Here's how the part is built. I have some questions about the finished solid (model axes, mm). A direction names the side the tool comes from. Give positions to 0.01 mm unless a question says otherwise; leave off trailing zeros. Write each loop counter-clockwise with the first axis right and the second up, starting at its lowest first coordinate (ties: lowest second). Pieces come first, ordered by that corner, then holes. Notation, with made-up numbers: (40, 58.5) - (70, 58.5) arc R36 ccw to (70, 92.5) - close; hole circle Ø11 at (-9, 82). An arc over 180 degrees is marked (long way). One line per item, written item: value. Start each with the question number.
1) I'm going to push a flat-ended pin straight in: P1, Ø4.5, axis at y = 0, z = 76.2, coming from the -X side. Where does the tip first touch, or does it pass through?
2) Imagine slicing it at A-A on z = -157.5. Write out the boundary of the cut face in (x, y) (3 decimals), plus the area to 3 significant figures.
3) Please list where these lines run through material, in increasing order: L1, parallel to Y at x = 8.5, z = 11.5 (3 decimals); L2, parallel to X at y = -7.25, z = -201 (3 decimals); L3, parallel to Y at x = -24, z = -76. Write a range as [from, to].
4) We'd pull the mould along Y, two halves only. Please class faces 1 (the flat face through (-22.225, 0, 3)), 2 (the flat face through (0, 9.525, 3)), 3 (the flat face through (0, 10, 222.25)), 4 (the flat face through (0, -12.7, 3)): +Y half, -Y half, draft (parallel to the pull), parting line (faces both ways), or undercut.
5) On a 3-axis mill with a long thin cutter (end or side, diameter ignored), from which of +Z, -Z, +X, -X, +Y, -Y can I reach the whole of each face in a straight line? I mean faces 5 (the flat face through (-25.4, 0, 3)), 6 (the flat face through (22.225, 0, 3)). Say none if no direction works.
from build123d import *

# Parameters (mm, degrees)
SKETCH1_W           = 50.8
SKETCH1_H           = 25.4
SKETCH1_W_2         = 44.45
SKETCH1_H_2         = 19.05
BOSS_EXTRUDE1_DEPTH = 222.25
SKETCH3_R           = 2.15265
SKETCH3_R_2         = 2.159
CUT_EXTRUDE2_DEPTH  = 51.8
SKETCH4_R           = 2.4892
CUT_EXTRUDE3_DEPTH  = 51.8
SKETCH5_R           = 2.4892
CUT_EXTRUDE4_DEPTH  = 26.4


with BuildPart() as part:
    # Sketch1 → Boss-Extrude1 (new body, symmetric)
    with BuildSketch(Plane.XY):
        Rectangle(SKETCH1_W, SKETCH1_H)
        Rectangle(SKETCH1_W_2, SKETCH1_H_2, mode=Mode.SUBTRACT)
    extrude(amount=BOSS_EXTRUDE1_DEPTH, both=True)

    # Sketch3 → Cut-Extrude2 (cut, through all)
    with BuildSketch(Plane(origin=(25.4, 0, 0), x_dir=(0, 0, -1), z_dir=(1, 0, 0))):
        with Locations((-215.9, 0)):
            Circle(SKETCH3_R)
        with Locations((-190.5, 0)):
            Circle(SKETCH3_R)
        with Locations((-165.1, 0)):
            Circle(SKETCH3_R)
        with Locations((215.9, 0)):
            Circle(SKETCH3_R_2)
        with Locations((190.5, 0)):
            Circle(SKETCH3_R_2)
        with Locations((165.1, 0)):
            Circle(SKETCH3_R_2)
    extrude(amount=-CUT_EXTRUDE2_DEPTH, mode=Mode.SUBTRACT)

    # Sketch4 → Cut-Extrude3 (cut, through all)
    with BuildSketch(Plane(origin=(25.4, 0, 0), x_dir=(0, 0, -1), z_dir=(1, 0, 0))):
        with Locations((-139.7, 0)):
            Circle(SKETCH4_R)
        with Locations((-127, 0)):
            Circle(SKETCH4_R)
        with Locations((-114.3, 0)):
            Circle(SKETCH4_R)
        with Locations((-101.6, 0)):
            Circle(SKETCH4_R)
        with Locations((-88.9, 0)):
            Circle(SKETCH4_R)
        with Locations((-76.2, 0)):
            Circle(SKETCH4_R)
        with Locations((-63.5, 0)):
            Circle(SKETCH4_R)
        with Locations((-50.8, 0)):
            Circle(SKETCH4_R)
        with Locations((-38.1, 0)):
            Circle(SKETCH4_R)
        with Locations((-25.4, 0)):
            Circle(SKETCH4_R)
        with Locations((-12.7, 0)):
            Circle(SKETCH4_R)
        Circle(SKETCH4_R)
        with Locations((12.7, 0)):
            Circle(SKETCH4_R)
        with Locations((25.4, 0)):
            Circle(SKETCH4_R)
        with Locations((38.1, 0)):
            Circle(SKETCH4_R)
        with Locations((50.8, 0)):
            Circle(SKETCH4_R)
        with Locations((63.5, 0)):
            Circle(SKETCH4_R)
        with Locations((76.2, 0)):
            Circle(SKETCH4_R)
        with Locations((88.9, 0)):
            Circle(SKETCH4_R)
        with Locations((101.6, 0)):
            Circle(SKETCH4_R)
        with Locations((114.3, 0)):
            Circle(SKETCH4_R)
        with Locations((127, 0)):
            Circle(SKETCH4_R)
        with Locations((139.7, 0)):
            Circle(SKETCH4_R)
    extrude(amount=-CUT_EXTRUDE3_DEPTH, mode=Mode.SUBTRACT)

    # Sketch5 → Cut-Extrude4 (cut, through all)
    with BuildSketch(Plane.XZ.offset(12.7)):
        with Locations((-12.7, 133.35)):
            Circle(SKETCH5_R)
        with Locations((0, 133.35)):
            Circle(SKETCH5_R)
        with Locations((12.7, 133.35)):
            Circle(SKETCH5_R)
        with Locations((12.7, -133.35)):
            Circle(SKETCH5_R)
        with Locations((0, -133.35)):
            Circle(SKETCH5_R)
        with Locations((-12.7, -133.35)):
            Circle(SKETCH5_R)
        with Locations((-12.7, 25.4)):
            Circle(SKETCH5_R)
        with Locations((12.7, 25.4)):
            Circle(SKETCH5_R)
        with Locations((12.7, 12.7)):
            Circle(SKETCH5_R)
        with Locations((-12.7, 12.7)):
            Circle(SKETCH5_R)
        with Locations((12.7, 0)):
            Circle(SKETCH5_R)
        with Locations((-12.7, 0)):
            Circle(SKETCH5_R)
        with Locations((12.7, -12.7)):
            Circle(SKETCH5_R)
        with Locations((-12.7, -12.7)):
            Circle(SKETCH5_R)
        with Locations((12.7, -25.4)):
            Circle(SKETCH5_R)
        with Locations((-12.7, -25.4)):
            Circle(SKETCH5_R)
        with Locations((12.7, -38.1)):
            Circle(SKETCH5_R)
        with Locations((-12.7, -38.1)):
            Circle(SKETCH5_R)
        with Locations((12.7, -50.8)):
            Circle(SKETCH5_R)
        with Locations((-12.7, -50.8)):
            Circle(SKETCH5_R)
        with Locations((12.7, -63.5)):
            Circle(SKETCH5_R)
        with Locations((-12.7, -63.5)):
            Circle(SKETCH5_R)
        with Locations((12.7, -76.2)):
            Circle(SKETCH5_R)
        with Locations((-12.7, -76.2)):
            Circle(SKETCH5_R)
    extrude(amount=-CUT_EXTRUDE4_DEPTH, mode=Mode.SUBTRACT)


solid = part.part
Numbers:
1. P1: through
2. outline: (-25.4, -12.7) - (25.4, -12.7) - (25.4, 12.7) - (-25.4, 12.7) - close; hole (-22.225, -9.525) - (22.225, -9.525) - (22.225, 9.525) - (-22.225, 9.525) - close
2. area: 444 mm^2
3. L1: [-12.7, -9.525], [9.525, 12.7]
3. L2: [-25.4, -22.225], [22.225, 25.4]
3. L3: [-12.7, -2.48], [2.48, 12.7]
4. face 1: undercut
4. face 2: undercut
4. face 3: draft
4. face 4: -Y half
5. face 5: +Z, -Z, -X, +Y, -Y
5. face 6: +Z, -Z
